Autodesk Inventor part; units mm, degrees
ref_plane "YZ Plane" through (0, 0, 0) normal (1, 0, 0) x (0, 1, 0)
ref_plane "XZ Plane" through (0, 0, 0) normal (0, 1, 0) x (-1, 0, 0)
ref_plane "XY Plane" through (0, 0, 0) normal (0, 0, 1) x (1, 0, 0)
sketch "スケッチ1" plane through (0, 0, 0) normal (0, 0, 1) x (1, 0, 0)
  line L0 (-14, 0) -> (14, 0)
  line L1 (14, 0) -> (14, 23)
  line L2 (14, 23) -> (-14, 23)
  line L3 (-14, 23) -> (-14, 0)
  circle A0 centre (-10, 18) radius 1.65
  circle A1 centre (10, 18) radius 1.65
  point P0 (0, 0)
  dimension "d0" = 3.3
  dimension "d1" = 3.3
  dimension "d2" = 0
  dimension "d3" = 20
  dimension "d4" = 18
  dimension "d5" = 10
  dimension "d6" = 23
  dimension "d7" = 28
  dimension "d8" = 14
  dimension "d9" = 0
extrude "押し出し1" add sketch "スケッチ1" along normal blind 1.6
sketch "スケッチ2" plane through (-14, 0, 0) normal (0, -1, 0) x (1, 0, 0)
  line L0 (0, 0) -> (28, 0)
  line L1 (28, 0) -> (28, 1.6)
  line L2 (0, 1.6) -> (28, 1.6)
  line L3 (0, 0) -> (0, 1.6)
  line L4 (-16, 3.25) -> (44, 3.25)
  line L5 (44, 3.25) -> (44, -1.75)
  line L6 (44, -1.75) -> (-16, -1.75)
  line L7 (-16, -1.75) -> (-16, 3.25)
  line L8 (11.5, 30.75) -> (16.5, 30.75)
  line L9 (16.5, 30.75) -> (16.5, -29.25)
  line L10 (16.5, -29.25) -> (11.5, -29.25)
  line L11 (11.5, -29.25) -> (11.5, 30.75)
  point P0 (14, 0)
  dimension "d12" = 60
  dimension "d13" = 60
  dimension "d14" = 5
  dimension "d15" = 5
  dimension "d16" = 1.75
  dimension "d17" = 2.5
  dimension "d18" = 30
  dimension "d19" = 29.25
extrude "押し出し2" add sketch "スケッチ2" along normal blind 1.4
sketch "スケッチ3" plane through (0, 0, 0) normal (1, 0, 0) x (0, 1, 0)
  line L0 (-1.4, 3.25) -> (0, 3.25)
  line L1 (0, 30.75) -> (0, 3.25)
  line L2 (0, 30.75) -> (-1.4, 30.75)
  line L3 (-1.4, 3.25) -> (-1.4, 30.75)
  line L4 (0, -1.75) -> (-1.4, -1.75)
  line L5 (-1.4, -29.25) -> (-1.4, -1.75)
  line L6 (0, -29.25) -> (-1.4, -29.25)
  line L7 (0, -1.75) -> (0, -29.25)
  line L8 (0, 0) -> (23, 0)
  line L9 (23, 0) -> (23, 1.6)
  line L10 (0, 1.6) -> (23, 1.6)
  line L11 (0, 0) -> (0, 1.6)
  line L12 (0, 11.6) -> (10, 1.6)
  line L13 (10, 0) -> (0, -10)
  line L14 (10, 0) -> (10, 1.6)
  line L15 (0, 1.6) -> (10, 1.6)
  line L16 (10, 0) -> (0, 0)
  line L17 (0, -10) -> (0, 0)
  line L18 (0, 1.6) -> (0, 11.6)
  dimension "d22" = 45
  dimension "d23" = 45
  dimension "d24" = 0
  dimension "d25" = 10
extrude "押し出し3" add sketch "スケッチ3" along normal mid plane 1.4 contours L1 L12 L10 L18
fillet "フィレット1" radius 4 2 edges at (-14, 23, 0.8) (14, 23, 0.8)
equation "\"d1\" = d0"
equation "\"d13\" = d12"
equation "\"d15\" = d14"
equation "\"d23\" = d22"
properties part number "thrust-checker"
Design review of the part built by this model. Coordinates are the model's own, in mm. A direction names the side the tool comes from. Give positions to 0.01 mm unless a question says otherwise; leave off trailing zeros. Loops run counter-clockwise (first coordinate to the right, second up) from the corner with the lowest first, then second, coordinate; pieces in that order, holes last. Notation, with made-up numbers: (47.25, 38) -> (52.25, 38) arc R6 cw to (52.25, 44) -> close; hole circle Ø1 at (49, 88.25). An arc over 180 degrees is marked (long way). One line per item, written item: value.
Q1. We need section C-C on y = 0.75. Give the boundary of the cut face in (x, z).
Numbers:
outline: (-14, 0) -> (14, 0) -> (14, 1.6) -> (0.7, 1.6) -> (0.7, 10.85) -> (-0.7, 10.85) -> (-0.7, 1.6) -> (-14, 1.6) -> close
Q2. We need section B-B on x = 5.5. Give the boundary of the cut face in (y, z).
Numbers:
outline: (-1.4, -1.75) -> (0, -1.75) -> (0, 0) -> (23, 0) -> (23, 1.6) -> (0, 1.6) -> (0, 3.25) -> (-1.4, 3.25) -> close
Q3. For pin 1 Ø1.3 at (y, z) = (11.5, 1) entering from -X; pin 2 Ø6 at (x, y) = (6.5, 10.5) entering from +Z; pin 3 Ø5 at (y, z) = (4.5, 5) entering from +X, all flat-tipped, find the tip position at first contact; note any pin that passes through.
Numbers:
pin 1: stops at x = -14
pin 2: stops at z = 1.6
pin 3: stops at x = 0.7
Q4. We need section A-A on y = 18. Give the boundary of the cut face in (x, z), and give its area (3 significant figures).
Numbers:
outline: (-14, 0) -> (-11.65, 0) -> (-11.65, 1.6) -> (-14, 1.6) -> close; (-8.35, 0) -> (8.35, 0) -> (8.35, 1.6) -> (-8.35, 1.6) -> close; (11.65, 0) -> (14, 0) -> (14, 1.6) -> (11.65, 1.6) -> close
area: 34.2 mm^2
Q5. For L1, parallel to Y at x = 10, z = 0.7; L2, parallel to Z at x = -6, y = 1.25; L3, parallel to X at y = 2, z = 9.5, list the stretches that pass through material, from the lowest coordinate up.
Numbers:
L1: y = -1.4 to 16.35, 19.65 to 23
L2: z = 0 to 1.6
L3: x = -0.7 to 0.7
Q6. Machinability: for faces 1 (the flat face through (-2.5, -1, -16)), 2 (the flat face through (0.7, 3, 4)), 3 (the flat face through (-0.7, 3, 4)), 4 (the flat face through (2.5, -1, -15)), which of the approach directions +Z, -Z, +X, -X, +Y, -Y give a long, thin tool a straight path to every point of the face, cutting with its end or side? Answer none if there is none.
Numbers:
face 1: -Z, -X, +Y, -Y
face 2: +Z, +X, +Y
face 3: +Z, -X, +Y
face 4: -Z, +X, +Y, -Y
Q7. Draft analysis for pull direction X (two halves, no side actions). For faces 5 (the cylindrical face through (-9.11, 16.61, 0.79)), 6 (the cylindrical face through (10.89, 16.61, 0.79)), 7 (the flat face through (0, 0, -1)), 8 (the flat face through (2.5, -1, 17)), state which applies: pulls with the +X half, pulls with the -X half, needs draft (parallel to the pull), parting line crosses it, or undercut.
Numbers:
face 5: undercut
face 6: undercut
face 7: needs draft
face 8: pulls with the +X half
Q8. We need section D-D on z = 26.5. Give the boundary of the cut face in (x, y), and give its area (3 significant figures).
Numbers:
outline: (-2.5, -1.4) -> (2.5, -1.4) -> (2.5, 0) -> (-2.5, 0) -> close
area: 7.00 mm^2
